Check sheet for the modelled part. Datum: model origin and axes. Units: mm. Face numbers are marked on the shaded views. A direction names the side the tool comes from. Coordinates: 2 decimals unless noted, no trailing zeros. Loops run counter-clockwise (first coordinate to the right, second up) from the corner with the lowest first, then second, coordinate; pieces in that order, holes last.
```python
from build123d import *

# Parameters (mm, degrees)
SKETCH1_W           = 23.6982
SKETCH1_H           = 16.7132
BOSS_EXTRUDE1_DEPTH = 6.096
SKETCH2_W           = 11.9888
SKETCH2_H           = 4.4704
BOSS_EXTRUDE2_DEPTH = 13.2588
SKETCH3_W           = 11.3792
SKETCH3_H           = 2.0574
CUT_EXTRUDE1_DEPTH  = 9.017
SKETCH4_R           = 3.048
BOSS_EXTRUDE3_DEPTH = 1.778
SKETCH5_R           = 2.5781
BOSS_EXTRUDE4_DEPTH = 1.8542


with BuildPart() as part:
    # Sketch1 → Boss-Extrude1 (new body)
    with BuildSketch(Plane(origin=(0, 0, 0), x_dir=(1, 0, 0), z_dir=(0, 1, 0))):
        with Locations((11.8491, 8.3566)):
            Rectangle(SKETCH1_W, SKETCH1_H)
    extrude(amount=BOSS_EXTRUDE1_DEPTH)

    # Sketch2 → Boss-Extrude2 (add)
    with BuildSketch(Plane.ZY):
        with Locations((-8.3566, 3.048)):
            Rectangle(SKETCH2_W, SKETCH2_H)
    extrude(amount=BOSS_EXTRUDE2_DEPTH)

    # Sketch3 → Cut-Extrude1 (cut)
    with BuildSketch(Plane.ZY.offset(13.2588)):
        with Locations((-8.3566, 2.1463)):
            Rectangle(SKETCH3_W, SKETCH3_H)
    extrude(amount=-CUT_EXTRUDE1_DEPTH, mode=Mode.SUBTRACT)

    # Sketch4 → Boss-Extrude3 (add)
    with BuildSketch(Plane.XY):
        with Locations((20.6502, 3.048)):
            Circle(SKETCH4_R)
    extrude(amount=BOSS_EXTRUDE3_DEPTH)

    # Sketch5 → Boss-Extrude4 (add)
    with BuildSketch(Plane.XY.offset(1.778)):
        with Locations((20.6502, 3.048)):
            Circle(SKETCH5_R)
    extrude(amount=BOSS_EXTRUDE4_DEPTH)


solid = part.part
```
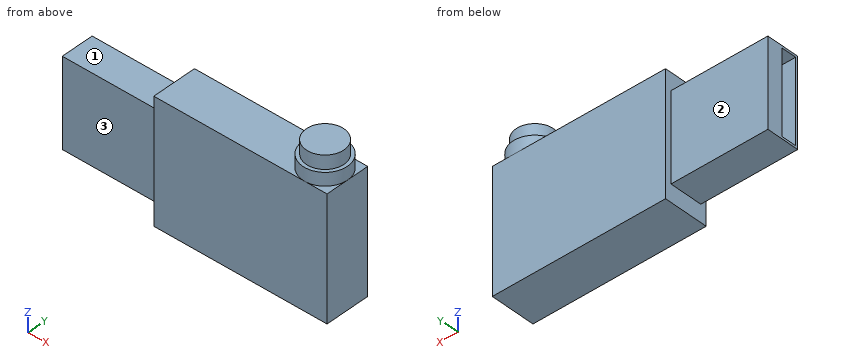
1) Depth check by flat-ended pin: pin 1 (2.5 mm diameter, centred on x = -7.5, y = 2.5, fed in from -Z); pin 2 (1.5 mm diameter, centred on x = 7.5, z = -7.5, fed in from -Y); pin 3 (4.5 mm diameter, centred on x = -9, z = -8.5, fed in from -Y); pin 4 (10 mm diameter, centred on x = -7, z = -8.5, fed in from +Y). Enter the tip coordinate at first touch or a pass-through.
Answer sheet:
pin 1: stops at z = -14.35
pin 2: stops at y = 0
pin 3: stops at y = 0.81
pin 4: stops at y = 5.28
2) Section check B-B on y = 3.75. Enter the section's corners in (x, z).
Answer sheet:
outline: (-13.26, -14.35) - (0, -14.35) - (0, -16.71) - (23.7, -16.71) - (23.7, 0) - (23.62, 0) - (23.62, 1.78) - (23.13, 1.78) - (23.13, 3.63) - (18.17, 3.63) - (18.17, 1.78) - (17.68, 1.78) - (17.68, 0) - (0, 0) - (0, -2.36) - (-13.26, -2.36) - close
3) Set-up check for the marked faces 1, 2 and 3: record each of +Z, -Z, +X, -X, +Y, -Y from which the full face is reachable in a straight line by a thin tool's end or side.
Answer sheet:
face 1: +Z, -X, +Y, -Y
face 2: +Z, -Z, -X, +Y
face 3: +Z, -Z, -X, -Y
4) Section check D-D on z = -1.5. Enter the section's corners in (x, y).
Answer sheet:
outline: (0, 0) - (23.7, 0) - (23.7, 6.1) - (0, 6.1) - close
5) Section check C-C on x = 20. Enter the section's corners in (y, z).
Answer sheet:
outline: (0, -16.71) - (6.1, -16.71) - (6.1, 0) - (6.03, 0) - (6.03, 1.78) - (5.54, 1.78) - (5.54, 3.63) - (0.55, 3.63) - (0.55, 1.78) - (0.07, 1.78) - (0.07, 0) - (0, 0) - close
6) Section check A-A on z = -6.75. Enter the section's corners in (x, y) (3 decimals).
Answer sheet:
outline: (-13.259, 0.813) - (0, 0.813) - (0, 0) - (23.698, 0) - (23.698, 6.096) - (0, 6.096) - (0, 5.283) - (-13.259, 5.283) - (-13.259, 3.175) - (-4.242, 3.175) - (-4.242, 1.118) - (-13.259, 1.118) - close
7) Scan lines: line 1 (Y direction, x = -8.5, z = -13) (3 decimals); line 2 (Z direction, x = 14, y = 1); line 3 (X direction, y = 5.5, z = -10.75). Record each from-to range of solid material in increasing order.
Answer sheet:
line 1: y = 0.813 to 1.118, 3.175 to 5.283
line 2: z = -16.71 to 0
line 3: x = 0 to 23.7
